Could you check a few things on this model? Use its own coordinates, in mm. A direction names the side the tool comes from. Coordinates: 2 decimals unless noted, no trailing zeros. Order: outer loops, then holes, each group sorted by start corner. A loop starts at its lowest first (then second) coordinate and runs counter-clockwise, first axis right, second up. Notation, with made-up numbers: (81.5, 55) -> (104.5, 55) arc R22 cw to (104.5, 92) -> close; hole circle Ø4 at (59.5, 40.5). An arc over 180 degrees is marked (long way). Put each result on its own line as item: value. Start each with the question number.
Q1. If we section it at D-D (z = 4.1): Count the separate pieces of the cut face and the enclosed holes in it, and give its area (3 significant figures).
Q2. If we section it at A-A (x = 54.15): Please give me the cut outline in (y, z).
Q3. We'd pull the mould along Y, two halves only. Please class faces 6 (the face through (-20.75, 0, 3)), 7 (the face through (22.5, -61, 3)), 8 (the face through (-51, 75, 3)): +Y half, -Y half, draft (parallel to the pull), parting line (faces both ways), or undercut.
Q4. If we section it at B-B (y = 59.5): Please give me the cut outline in (x, z).
Q5. If we section it at C-C (x = -73.5): Please give me the cut outline in (y, z), and give its area (3 significant figures).
Q6. For faces 1 (the face through (-34, 53, 3)), 2 (the face through (-30.5, -61, 3)), 3 (the face through (93.992, -1.216, 2.958)), 4 (the face through (-93.992, 1.216, 2.958)), 5 (the face through (-22.5, 61, 3)), which set-ups out of +Z, -Z, +X, -X, +Y, -Y let a thin tool reach every point of the face, with its end or its side?
Q7. Please list where these lines run through material, in increasing order: line 1 along Y through (x, z) = (54.15, 4); line 2 along Y through (x, z) = (-20, 4.55); line 3 along Y through (x, z) = (-24.3, 2.9) (3 decimals).
Q8. Will these pins go through, and if not, where does the flat tip stop? pin 1 (1.8 mm diameter, centred on x = -39, z = 2.5, fed in from -Y); pin 2 (3 mm diameter, centred on y = -70, z = 4, fed in from -X); pin 3 (1.8 mm diameter, centred on y = 69, z = 3, fed in from -X) (3 decimals).
from build123d import *

# Parameters (mm, degrees)
SKETCH8_R               = 1.5
SKETCH8_W               = 41.5
SKETCH8_H               = 21.5
BOSS_EXTRUDE1_DEPTH     = 6
SKETCH10_R              = 4
CUT_EXTRUDE2_DEPTH      = 1
CUT_EXTRUDE2_DEPTH_BACK = 7


with BuildPart() as part:
    # Sketch8 → Boss-Extrude1 (new body)
    with BuildSketch(Plane.XY):
        with BuildLine():
            Line((-56.665686266, -75), (-46, -75))
            Line((-46, -75), (-46, -65))
            Line((-46, -65), (-30.5, -65))
            Line((-30.5, -65), (-30.5, -57.029309822))
            Line((-30.5, -57.029309822), (-34, -57.029309822))
            Line((-34, -57.029309822), (-34, -49.029309822))
            Line((-34, -49.029309822), (-19, -49.029309822))
            Line((-19, -49.029309822), (-19, -57.029309822))
            Line((-19, -57.029309822), (-22.5, -57.029309822))
            Line((-22.5, -57.029309822), (-22.5, -65))
            Line((-22.5, -65), (22.5, -65))
            Line((22.5, -65), (22.5, -57.029309822))
            Line((22.5, -57.029309822), (19, -57.029309822))
            Line((19, -57.029309822), (19, -49.029309822))
            Line((19, -49.029309822), (34, -49.029309822))
            Line((34, -49.029309822), (34, -57.029309822))
            Line((34, -57.029309822), (30.5, -57.029309822))
            Line((30.5, -57.029309822), (30.5, -65))
            Line((30.5, -65), (46, -65))
            Line((46, -65), (46, -75))
            Line((46, -75), (56.665686266, -75))
            ThreePointArc((56.665686266, -75), (94, 0), (56.665686266, 75))
            Line((56.665686266, 75), (46, 75))
            Line((46, 75), (46, 65))
            Line((46, 65), (30.5, 65))
            Line((30.5, 65), (30.5, 57.029309822))
            Line((30.5, 57.029309822), (34, 57.029309822))
            Line((34, 57.029309822), (34, 49.029309822))
            Line((34, 49.029309822), (19, 49.029309822))
            Line((19, 49.029309822), (19, 57.029309822))
            Line((19, 57.029309822), (22.5, 57.029309822))
            Line((22.5, 57.029309822), (22.5, 65))
            Line((22.5, 65), (-22.5, 65))
            Line((-22.5, 65), (-22.5, 57.029309822))
            Line((-22.5, 57.029309822), (-19, 57.029309822))
            Line((-19, 57.029309822), (-19, 49.029309822))
            Line((-19, 49.029309822), (-34, 49.029309822))
            Line((-34, 49.029309822), (-34, 57.029309822))
            Line((-34, 57.029309822), (-30.5, 57.029309822))
            Line((-30.5, 57.029309822), (-30.5, 65))
            Line((-30.5, 65), (-46, 65))
            Line((-46, 65), (-46, 75))
            Line((-46, 75), (-56.665686266, 75))
            ThreePointArc((-56.665686266, 75), (-94, 0), (-56.665686266, -75))
        make_face()
        with Locations((-24.3, -4.875)):
            Circle(SKETCH8_R, mode=Mode.SUBTRACT)
        with Locations((-24.3, 4.875)):
            Circle(SKETCH8_R, mode=Mode.SUBTRACT)
        with Locations((24.3, 4.875)):
            Circle(SKETCH8_R, mode=Mode.SUBTRACT)
        with Locations((24.3, -4.875)):
            Circle(SKETCH8_R, mode=Mode.SUBTRACT)
        Rectangle(SKETCH8_W, SKETCH8_H, mode=Mode.SUBTRACT)
    extrude(amount=BOSS_EXTRUDE1_DEPTH)

    # Sketch10 → Cut-Extrude2 (cut, two sides)
    with BuildSketch(Plane.XY.offset(6)) as cut_extrude2_sk:
        with Locations((54.15, -34.722964698)):
            Circle(SKETCH10_R)
        with Locations((54.15, 33.277035302)):
            Circle(SKETCH10_R)
        with Locations((-45.21, -0.722964698)):
            Circle(SKETCH10_R)
    extrude(amount=CUT_EXTRUDE2_DEPTH, mode=Mode.SUBTRACT)
    extrude(cut_extrude2_sk.sketch, amount=-CUT_EXTRUDE2_DEPTH_BACK, mode=Mode.SUBTRACT)


solid = part.part
The answers:
1. separate pieces: 1
1. enclosed holes: 8
1. area: 21,200 mm^2
2. outline: (-75, 0) -> (-38.72, 0) -> (-38.72, 6) -> (-75, 6) -> close; (-30.72, 0) -> (29.28, 0) -> (29.28, 6) -> (-30.72, 6) -> close; (37.28, 0) -> (75, 0) -> (75, 6) -> (37.28, 6) -> close
3. face 6: undercut
3. face 7: draft
3. face 8: +Y half
4. outline: (-72.77, 0) -> (-30.5, 0) -> (-30.5, 6) -> (-72.77, 6) -> close; (-22.5, 0) -> (22.5, 0) -> (22.5, 6) -> (-22.5, 6) -> close; (30.5, 0) -> (72.77, 0) -> (72.77, 6) -> (30.5, 6) -> close
5. outline: (-58.6, 0) -> (58.6, 0) -> (58.6, 6) -> (-58.6, 6) -> close
5. area: 703 mm^2
6. face 1: +Z, -Z
6. face 2: +Z, -Z, -Y
6. face 3: +Z, -Z, +X
6. face 4: +Z, -Z, -X
6. face 5: +Z, -Z, +Y
7. line 1: -75 to -38.72, -30.72 to 29.28, 37.28 to 75
7. line 2: -65 to -57.03, -49.03 to -10.75, 10.75 to 49.03, 57.03 to 65
7. line 3: -49.029 to -6.375, -3.375 to 3.375, 6.375 to 49.029
8. pin 1: y = -65
8. pin 2: x = -64.37
8. pin 3: x = -64.795
